Could you check a few things on this model? Use its own coordinates, in mm. A direction names the side the tool comes from. Give positions to 0.01 mm unless a question says otherwise; leave off trailing zeros. Loops run counter-clockwise (first coordinate to the right, second up) from the corner with the lowest first, then second, coordinate; pieces in that order, holes last. Notation, with made-up numbers: (28, -12.5) - (64, -12.5) arc R29 ccw to (64, 25.5) - close; hole circle Ø3 at (-13.75, -9.75). An arc over 180 degrees is marked (long way). Use CSV: the item, a comma, the result in double quotes.
Autodesk Inventor part; units mm, degrees
ref_plane "Work Plane1" through (-47, 34, 13) normal (1, 0, 0) x (0, 0, -1)
ref_plane "Work Plane3" through (-47, -5, 13) normal (0, 1, 0) x (1, 0, 0)
ref_plane "YZ Plane" through (0, 0, 0) normal (1, 0, 0) x (0, 1, 0)
sketch "Sketch1" plane through (0, 0, 0) normal (0, 0, 1) x (1, 0, 0)
  line L0 (0, 0) -> (-53, 0)
  line L1 (-53, 0) -> (-53, 18)
  line L2 (-53, 18) -> (0, 18) construction
  line L3 (-53, 18) -> (-56, 18)
  line L4 (-56, 18) -> (-56, -3)
  line L5 (-56, -3) -> (0, -3)
  line L6 (0, -3) -> (0, 0)
  dimension "d0" = 18
  dimension "d1" = 3
  dimension "d2" = 3
  dimension "d3" = 56
extrude "Extrusion1" add sketch "Sketch1" along normal blind 10
mirror "Mirror1" about plane through (-34.1948, 1.3052, 0) normal (0, 0, -1) of "Extrusion1"
mirror "Mirror2" about plane through (-53, 18, 0) normal (0, 1, 0) of "Extrusion1", "Mirror1"
sketch "Sketch4" plane through (0, -3, -10) normal (0, 0, -1) x (-1, 0, 0)
  line L0 (0, 3) -> (53, 3)
  line L1 (0, 0) -> (0, 3)
  line L2 (56, 0) -> (0, 0)
  line L3 (56, 42) -> (56, 0)
  line L4 (56, 42) -> (0, 42)
  line L5 (0, 42) -> (0, 39)
  line L6 (0, 39) -> (53, 39)
  line L7 (53, 39) -> (53, 3)
  line L8 (0, 3) -> (53, 3)
  line L9 (0, 0) -> (0, 3)
  line L10 (56, 0) -> (0, 0)
  line L11 (56, 42) -> (56, 0)
  line L12 (56, 42) -> (0, 42)
  line L13 (0, 42) -> (0, 39)
  line L14 (0, 39) -> (53, 39)
  line L15 (53, 39) -> (53, 3)
extrude "Extrusion4" add sketch "Sketch4" along normal blind 5
mirror "Mirror3" about plane through (0, 0, 0) normal (0, 0, 1) of "Extrusion4"
sketch "Sketch11" plane through (-56, -3, -15) normal (0, -1, 0) x (1, 0, 0)
  line L0 (56, 0) -> (56, 30)
  line L1 (56, 30) -> (0, 30)
  line L2 (0, 0) -> (0, 30)
  line L3 (56, 0) -> (0, 0)
  line L4 (56, 0) -> (56, 30)
  line L5 (56, 30) -> (0, 30)
  line L6 (0, 0) -> (0, 30)
  line L7 (56, 0) -> (0, 0)
  point P0 (56, 15)
extrude "Extrusion11" cut sketch "Sketch11" against normal blind 10
sketch "Sketch13" plane through (0, 36, -15) normal (1, 0, 0) x (0, 0, -1)
  line L0 (-30, 3) -> (-28, 3)
  line L1 (-28, 3) -> (-28, -29)
  line L2 (-28, -29) -> (-30, -29)
  line L3 (-30, -29) -> (-30, 3)
  line L4 (-30, -29) -> (0, -29)
  point P0 (-15, -36)
  dimension "d65" = 2
extrude "Extrusion13" cut sketch "Sketch13" against normal up to next
mirror "Mirror4" about plane through (0, 0, 0) normal (0, 0, 1) of "Extrusion13"
sketch "Sketch14" plane through (-56, 7, 13) normal (-1, 0, 0) x (0, 0, 1)
  line L0 (-26, 32) -> (-26, 0)
  line L1 (-26, 0) -> (0, 0)
  line L2 (0, 32) -> (-26, 32)
  circle A0 centre (-13, 10) radius 6.5 construction
  line L3 (-13, 10) -> (-26, 10) construction
  line L4 (-13, 10) -> (-13, 32) construction
  circle A1 centre (-13, 10) radius 1.5
  circle A2 centre (-13, 16.5) radius 1.5
  point P0 (-13, -7)
  point P1 (-13, 0)
  dimension "d68" = 13
  dimension "d69" = 22
  dimension "d71" = 3
  dimension "d72" = 3
extrude "Extrusion14" cut sketch "Sketch14" against normal up to next
pattern_circular "Circular Pattern6" count 4 over 360 about axis through (-56, 17, 0) along (1, 0, 0) of "Extrusion14"
sketch "Sketch15" plane through (-53, 36, 13) normal (0, -1, 0) x (1, 0, 0)
  line L0 (53, -26) -> (53, 0)
  line L1 (53, 0) -> (0, 0)
  circle A0 centre (37, -13) radius 6.5 construction
  line L2 (37, -13) -> (37, 0) construction
  circle A1 centre (37, -6.5) radius 1.5
  circle A2 centre (37, -13) radius 1.5
  point P0 (53, -13)
  point P1 (53, -13)
  dimension "d78" = 13
  dimension "d79" = 16
  dimension "d80" = 3
  dimension "d81" = 3
extrude "Extrusion15" cut sketch "Sketch15" against normal up to next
pattern_circular "Circular Pattern7" count 4 over 360 about axis through (-16, 36, 0) along (0, 1, 0) of "Extrusion15"
sketch "Sketch16" plane through (-56, 7, -15) normal (0, -1, 0) x (1, 0, 0)
  line L0 (0, 2) -> (3, 2)
  line L1 (3, 28) -> (3, 2)
  line L2 (3, 28) -> (0, 28)
  line L3 (0, 2) -> (0, 28)
  line L4 (0, 2) -> (3, 2)
  line L5 (3, 28) -> (3, 2)
  line L6 (3, 28) -> (0, 28)
  line L7 (0, 2) -> (0, 28)
  point P0 (56, 15)
extrude "Extrusion16" add sketch "Sketch16" along normal blind 14
ref_plane "Work Plane1" through (-47, 34, 13) normal (1, 0, 0) x (0, 0, -1)
sketch "Sketch17" plane through (-47, 34, 13) normal (1, 0, 0) x (0, 0, -1)
  line L0 (0, 0) -> (0, -41)
  line L1 (26, -41) -> (0, -41)
  line L2 (0, -41) -> (0, -39)
  line L3 (0, -39) -> (26, -39)
  line L4 (26, -39) -> (26, -41)
  point P0 (13, -34)
  dimension "d92" = 2
extrude "Extrusion17" add sketch "Sketch17" along normal blind 40
ref_plane "Work Plane3" through (-47, -5, 13) normal (0, 1, 0) x (1, 0, 0)
sketch "Sketch18" plane through (-47, -5, 13) normal (0, 1, 0) x (1, 0, 0)
  circle A0 centre (31, 13) radius 1.5
  circle A1 centre (31, 13) radius 2
  point P0 (47, 13)
  dimension "d95" = 4
extrude "Extrusion18" cut sketch "Sketch18" against normal up to next contours A0 | A1
sketch "Sketch23" plane through (0, 36, 13) normal (0, 0, 1) x (1, 0, 0)
  line L0 (0, 0) -> (-53, 0)
  line L1 (-56, 3) -> (0, 3)
  line L2 (-56, -43) -> (-56, 3)
  line L3 (-7, -43) -> (-56, -43)
  line L4 (-47, -41) -> (-7, -41)
  line L5 (-53, 0) -> (-53, -43)
  line L6 (0, 0) -> (-53, 0)
  line L7 (0, 3) -> (0, 0)
  line L8 (-56, 3) -> (0, 3)
  line L9 (-56, -43) -> (-56, 3)
  line L10 (-53, -43) -> (-56, -43)
  line L11 (0, 0) -> (-56, 0)
  line L12 (-56, 0) -> (-56, 4.5)
  line L13 (-56, 4.5) -> (0, 4.5)
  line L14 (0, 4.5) -> (0, 0)
  line L15 (-7, -41) -> (-56, -41)
  line L16 (-56, -41) -> (-56, -45.5)
  line L17 (-56, -45.5) -> (-7, -45.5)
  line L18 (-7, -45.5) -> (-7, -41)
  point P0 (0, -36)
  dimension "d110" = 3
  dimension "d111" = 2
  dimension "d112" = 1.5
  dimension "d113" = 2.5
sketch "Sketch24" plane through (-56, 39, 13) normal (0, 1, 0) x (1, 0, 0)
  circle A0 centre (40, 19.5) radius 1.5
  circle A1 centre (46.5, 13) radius 1.5
  circle A2 centre (33.5, 13) radius 1.5
  circle A3 centre (40, 6.5) radius 1.5
  circle A4 centre (40, 13) radius 1.5
  line L0 (56, 26) -> (0, 26)
  line L1 (0, 0) -> (0, 26)
  line L2 (0, 0) -> (56, 0)
  line L3 (56, 0) -> (56, 26)
  point P0 (56, 13)
  dimension "d114" = 26
extrude "Extrusion22" add sketch "Sketch23" against normal up to surface (26 mm away) contours L0 L11 L2 L1 L7 | L1 L12 L13 L14 | L15 L4 L18 L3 L5 | L5 L3 L2 L15 | L3 L18 L17 L16
sketch "Sketch25" plane through (-53, 36, 13) normal (0, 0, 1) x (1, 0, 0)
  line L0 (-3, 4.5) -> (-3, -45.5)
  line L1 (-3, -45.5) -> (46, -45.5)
  line L2 (46, -41) -> (46, -45.5)
  line L3 (46, -41) -> (0, -41)
  line L4 (0, 0) -> (0, -41)
  line L5 (53, 0) -> (0, 0)
  line L6 (53, 4.5) -> (53, 0)
  line L7 (53, 4.5) -> (-3, 4.5)
  point P0 (53, -36)
  dimension "d117" = 3
sketch "Sketch26" plane through (-56, -9.5, -13) normal (-1, 0, 0) x (0, 0, 1)
  line L0 (0, 0) -> (0, 50)
  line L1 (26, 0) -> (0, 0)
  line L2 (26, 50) -> (26, 0)
  line L3 (26, 50) -> (0, 50)
  circle A0 centre (13, 20) radius 1.5
  circle A1 centre (19.5, 26.5) radius 1.5
  circle A2 centre (6.5, 26.5) radius 1.5
  circle A3 centre (13, 26.5) radius 1.5
  circle A4 centre (13, 33) radius 1.5
  line L4 (0, 0) -> (0, 50)
  line L5 (26, 0) -> (0, 0)
  line L6 (26, 50) -> (26, 0)
  circle A5 centre (13, 20) radius 1.5
  circle A6 centre (19.5, 26.5) radius 1.5
  circle A7 centre (6.5, 26.5) radius 1.5
  circle A8 centre (13, 26.5) radius 1.5
  circle A9 centre (13, 33) radius 1.5
  line L7 (26, 50) -> (0, 50)
  point P0 (13, 9.5)
extrude "Extrusion23" add sketch "Sketch26" along normal blind 2
sketch "Sketch27" plane through (0, 40.5, 13) normal (0, 1, 0) x (1, 0, 0)
  line L0 (-58, 26) -> (0, 26)
  line L1 (0, 0) -> (0, 26)
  circle A0 centre (-16, 13) radius 6.5 construction
  circle A1 centre (-16, 19.5) radius 1.5
  circle A2 centre (-16, 13) radius 1.5
  line L2 (-16, 13) -> (0, 13) construction
  line L3 (-16, 13) -> (-16, 26) construction
  dimension "d121" = 13
  dimension "d120" = 3
  dimension "d122" = 3
  dimension "d123" = 16
extrude "Extrusion24" cut sketch "Sketch27" against normal up to surface (4.5 mm away)
pattern_circular "Circular Pattern8" count 4 over 360 about axis through (-16, 40.5, 0) along (0, -1, 0) of "Extrusion24"
sketch "Sketch28" plane through (-53, -5, 13) normal (0, 1, 0) x (1, 0, 0)
  circle A0 centre (37, 13) radius 1.5
  circle A1 centre (37, 13) radius 2
  point P0 (53, 13)
  dimension "d129" = 4
extrude "Extrusion25" cut sketch "Sketch28" against normal up to next contours A0 | A1
sketch "Sketch29" plane through (-58, -9.5, -13) normal (-1, 0, 0) x (0, 0, 1)
  line L0 (0, 50) -> (0, 0)
  line L1 (26, 0) -> (26, 50)
  line L2 (26, 50) -> (0, 50)
  line L3 (26, 45.5) -> (0, 45.5)
  point P0 (13, 9.5)
extrude "Extrusion26" add sketch "Sketch29" along normal blind 79.25
sketch "Sketch30" plane through (0, 40.5, 13) normal (0, 1, 0) x (1, 0, 0)
  line L0 (-137.25, 26) -> (0, 26)
  line L1 (-137.25, 0) -> (-137.25, 26)
  line L2 (0, 0) -> (-137.25, 0)
  arc A0 (-137.25, 13) -> (-68.625, 0) centre (-68.625, 187.6304) ccw
  arc A1 (-68.625, 26) -> (-137.25, 13) centre (-68.625, -161.6304) ccw
  point P0 (0, 13)
extrude "Extrusion27" cut sketch "Sketch30" against normal up to next
fillet "Fillet9" radius 3 1 edges at (-137.25, 38.25, 0)
fillet "Fillet10" radius 10 1 edges at (-58, 36, 0)
fillet "Fillet11" radius 10 1 edges at (-53, 36, 0)
fillet "Fillet12" radius 5 1 edges at (-58, -9.5, 0)
fillet "Fillet13" radius 2 4 edges at (0, 40.5, 0) (0, 36, 0) (-7, -9.5, 0) (-7, -5, 0)
fillet "Fillet14" radius 10 1 edges at (-53, -5, 0)
equation "\"d72\" = d71"
properties part number "CLAW"
1) Suppose I cut it at B-B (x = -22.5). Please give me the cut outline in (y, z).
Answer below:
outline,"(-9.5, -13) - (-5, -13) - (-5, 13) - (-9.5, 13) - close; (36, -13) - (40.5, -13) - (40.5, -1.5) - (36, -1.5) - close; (36, 1.5) - (40.5, 1.5) - (40.5, 13) - (36, 13) - close"
2) Which directions (+Z, -Z, +X, -X, +Y, -Y) give clear straight access to the entire face, cutting with the end or side of a thin tool? Please do faces 4 (the flat face through (-31, -9.5, 0)), 5 (the flat face through (-54, 21, -13)), 6 (the flat face through (-53, 13, 0)), 7 (the flat face through (-58, 11, -3)), 8 (the cylindrical face through (-17.5, 38.28, -6.57)).
Answer below:
face 4,"+Z, -Z, +X, -X, -Y"
face 5,"-Z, +X, -X, +Y, -Y"
face 6,"+Z, -Z, +X"
face 7,"+Z, -Z, -X, -Y"
face 8,"+Y"
3) We'd pull the mould along X, two halves only. Please class faces 1 (the cylindrical face through (-131.563, 38.282, -0.052)), 2 (the cylindrical face through (-14.5, 38.28, 6.57)), 3 (the flat face through (-92, 36, 0)): +X half, -X half, draft (parallel to the pull), parting line (faces both ways), or undercut.
Answer below:
face 1,"-X half"
face 2,"undercut"
face 3,"draft"
4) I'm going to push flat-ended pins straight in: P1, Ø1.8, axis at y = 17, z = 0, coming from the -X side; P2, Ø2.5, axis at x = -9.5, z = 0, coming from the +Y side; P3, Ø5, axis at y = 23.5, z = 0, coming from the -X side; P4, Ø13, axis at x = -112.5, z = -4, coming from the -Y side. Where does each tip first touch, or does it pass through?
Answer below:
P1,"passes through"
P2,"stops at y = -5"
P3,"stops at x = -58"
P4,"stops at y = 36"
5) Suppose I cut it at A-A (y = 17). Please give me the cut outline in (x, z), plus the area to 3 significant figures.
Answer below:
outline,"(-58, -13) - (-53, -13) - (-53, -8) - (-58, -8) - close; (-58, -5) - (-53, -5) - (-53, -1.5) - (-58, -1.5) - close; (-58, 1.5) - (-53, 1.5) - (-53, 5) - (-58, 5) - close; (-58, 8) - (-53, 8) - (-53, 13) - (-58, 13) - close"
area,"85.0 mm2"
6) Suppose I cut it at C-C (z = -6.5). Please give me the cut outline in (x, y), plus the area to 3 significant figures.
Answer below:
outline,"(-117.58, 36) - (-68, 36) arc R10 cw to (-58, 26) - (-58, 18.5) - (-53, 18.5) - (-53, 26) arc R10 cw to (-43, 36) - (-17.5, 36) - (-17.5, 40.5) - (-117.58, 40.5) - close; (-58, -4.5) arc R5 ccw to (-53, -9.5) - (-9, -9.5) arc R2 ccw to (-7, -7.5) - (-7, -7) arc R2 ccw to (-9, -5) - (-43, -5) arc R10 cw to (-53, 5) - (-53, 15.5) - (-58, 15.5) - close; (-14.5, 36) - (-2, 36) arc R2 ccw to (0, 38) - (0, 38.5) arc R2 ccw to (-2, 40.5) - (-14.5, 40.5) - close"
area,"991 mm2"
7) I need wall thicknesses on line 1 along Z through (x, y) = (-16, 38.8); line 2 along Y through (x, z) = (-24.5, -8.5); line 3 along Z through (x, y) = (-57.1, 10.5). Which ranges of each line are inside material? Lowest first, please.
Answer below:
line 1,"z = -13 to -8, -5 to -1.5, 1.5 to 5, 8 to 13"
line 2,"y = -9.5 to -5, 36 to 40.5"
line 3,"z = -13 to -1.5, 1.5 to 13"
8) Suppose I cut it at D-D (y = 23.5). Please give me the cut outline in (x, z), plus the area to 3 significant figures.
Answer below:
outline,"(-58, -13) - (-53, -13) - (-53, -1.5) - (-58, -1.5) - close; (-58, 1.5) - (-53, 1.5) - (-53, 13) - (-58, 13) - close"
area,"115 mm2"
